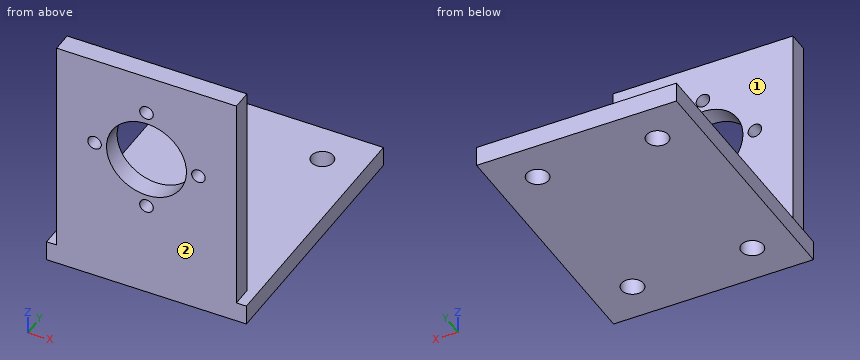
from build123d import *

# Parameters (mm, degrees)
SKETCH1_W           = 65
SKETCH1_H           = 50
BOSS_EXTRUDE1_DEPTH = 5
BOSS_EXTRUDE2_DEPTH = 55
SKETCH3_R           = 10
CUT_EXTRUDE1_DEPTH  = 92.923881554
SKETCH5_R           = 1.7
CUT_EXTRUDE2_DEPTH  = 92.923881554
SKETCH6_R           = 2.75
CUT_EXTRUDE3_DEPTH  = 69.60211367


with BuildPart() as part:
    # Sketch1 → Boss-Extrude1 (new body)
    with BuildSketch(Plane(origin=(0, 0, 0), x_dir=(0, 1, 0), z_dir=(0, 0, 1))):
        Rectangle(SKETCH1_W, SKETCH1_H)
    extrude(amount=BOSS_EXTRUDE1_DEPTH)

    # Sketch2 → Boss-Extrude2 (add)
    with BuildSketch(Plane.XY.offset(5)):
        Polygon((0, -32.5), (-22.5, -32.5), (-22.5, -27.5), (22.5, -27.5), (22.5, -32.5), align=None)
    extrude(amount=BOSS_EXTRUDE2_DEPTH)

    # Sketch3 → Cut-Extrude1 (cut, through all)
    with BuildSketch(Plane.XZ.offset(32.5)):
        with Locations(Location((0, 37, 0), (0, 0, 270))):
            Circle(SKETCH3_R)
    extrude(amount=-CUT_EXTRUDE1_DEPTH, mode=Mode.SUBTRACT)

    # Sketch5 → Cut-Extrude2 (cut, through all)
    with BuildSketch(Plane.XZ.offset(32.5)):
        with Locations(Location((0, 50, 0), (0, 0, 270))):
            Circle(SKETCH5_R)
        with Locations(Location((13, 37, 0), (0, 0, 270))):
            Circle(SKETCH5_R)
        with Locations(Location((0, 24, 0), (0, 0, 270))):
            Circle(SKETCH5_R)
        with Locations(Location((-13, 37, 0), (0, 0, 270))):
            Circle(SKETCH5_R)
    extrude(amount=-CUT_EXTRUDE2_DEPTH, mode=Mode.SUBTRACT)

    # Sketch6 → Cut-Extrude3 (cut, through all)
    with BuildSketch(Plane.XY.offset(5)):
        with Locations((-15, 22.5)):
            Circle(SKETCH6_R)
        with Locations((15, 22.5)):
            Circle(SKETCH6_R)
        with Locations((-15, -22.5)):
            Circle(SKETCH6_R)
        with Locations((15, -22.5)):
            Circle(SKETCH6_R)
    extrude(amount=-CUT_EXTRUDE3_DEPTH, mode=Mode.SUBTRACT)


solid = part.part
The listing builds one solid part. Answer for the finished solid, in the listing's coordinates (mm). Face numbers are marked on the shaded views. A direction names the side the tool comes from. Give positions to 0.01 mm unless a question says otherwise; leave off trailing zeros. Write each loop counter-clockwise with the first axis right and the second up, starting at its lowest first coordinate (ties: lowest second). Pieces come first, ordered by that corner, then holes.
Item 1: Section D-D, the plane x = 21.5 is taken. Write down the section's boundary in (y, z), plus the area to 3 significant figures.
Item 2: Which of the six approach directions +Z, -Z, +X, -X, +Y, -Y give full straight-line access (tool end or side, diameter ignored) to the marked faces 1 and 2?
Item 3: Section B-B, the plane x = -9 is taken. Write down the section's boundary in (y, z), plus the area to 3 significant figures.
Item 4: Find the intervals of material crossed by line 1 along Y through (x, z) = (-15, 2); line 2 along X through (y, z) = (-31.5, 24); line 3 along Y through (x, z) = (-9, 6), in increasing order.
Item 5: Section A-A, the plane z = 37 is taken. Write down the section's boundary in (x, y), plus the area to 3 significant figures.
Item 6: Section C-C, the plane y = -24 is taken. Write down the section's boundary in (x, z).
Item 7: Flat-ended cylindrical pins translate along their axes: P1, Ø4.5, axis at x = 15, y = -22.5, coming from the +Z side; P2, Ø9, axis at x = -15, y = 22.5, coming from the +Z side; P3, Ø4.5, axis at x = 0, z = 50, coming from the -Y side; P4, Ø1.5, axis at x = 11.5, z = 6.5, coming from the +Y side. Find the tip coordinate at first contact, or state that the pin passes through.
Completed:
1. outline: (-32.5, 0) - (32.5, 0) - (32.5, 5) - (-27.5, 5) - (-27.5, 60) - (-32.5, 60) - close
1. area: 600 mm2
2. face 1: +Z, +X, -X, +Y
2. face 2: +Z, -Z, +X, -X, -Y
3. outline: (-32.5, 0) - (32.5, 0) - (32.5, 5) - (-27.5, 5) - (-27.5, 32.64) - (-32.5, 32.64) - close; (-32.5, 41.36) - (-27.5, 41.36) - (-27.5, 60) - (-32.5, 60) - close
3. area: 556 mm2
4. line 1: y = -32.5 to -25.25, -19.75 to 19.75, 25.25 to 32.5
4. line 2: x = -22.5 to -1.7, 1.7 to 22.5
4. line 3: y = -32.5 to -27.5
5. outline: (-22.5, -32.5) - (-14.7, -32.5) - (-14.7, -27.5) - (-22.5, -27.5) - close; (-11.3, -32.5) - (-10, -32.5) - (-10, -27.5) - (-11.3, -27.5) - close; (10, -32.5) - (11.3, -32.5) - (11.3, -27.5) - (10, -27.5) - close; (14.7, -32.5) - (22.5, -32.5) - (22.5, -27.5) - (14.7, -27.5) - close
5. area: 91.0 mm2
6. outline: (-25, 0) - (-17.3, 0) - (-17.3, 5) - (-25, 5) - close; (-12.7, 0) - (12.7, 0) - (12.7, 5) - (-12.7, 5) - close; (17.3, 0) - (25, 0) - (25, 5) - (17.3, 5) - close
7. P1: passes through
7. P2: stops at z = 5
7. P3: stops at y = -32.5
7. P4: stops at y = -27.5
